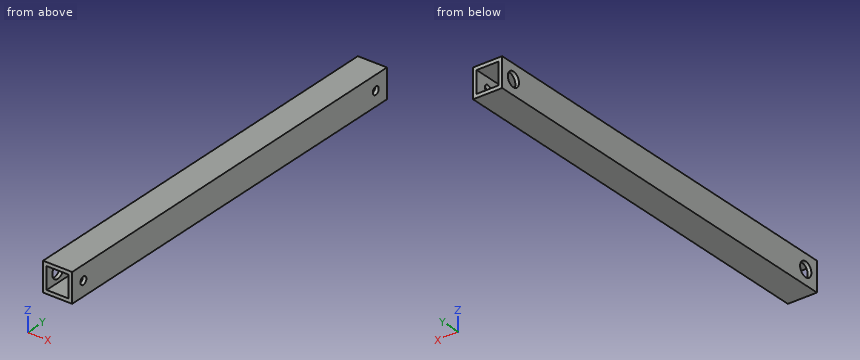
from build123d import *

# Parameters (mm, degrees)
SKETCH1_W           = 25.4
SKETCH1_H           = 25.4
SKETCH1_W_2         = 19.05
SKETCH1_H_2         = 19.05
BOSS_EXTRUDE1_DEPTH = 355.6
SKETCH2_R           = 3.3734375
CUT_EXTRUDE1_DEPTH  = 358.409680899
CUT_EXTRUDE2_REACH  = 359.41
SKETCH3_R           = 6.35


with BuildPart() as part:
    # Sketch1 → Boss-Extrude1 (new body)
    with BuildSketch(Plane(origin=(0, 0, 0), x_dir=(1, 0, 0), z_dir=(0, 1, 0))):
        with Locations((12.7, 12.7)):
            Rectangle(SKETCH1_W, SKETCH1_H)
        with Locations((12.7, 12.7)):
            Rectangle(SKETCH1_W_2, SKETCH1_H_2, mode=Mode.SUBTRACT)
    extrude(amount=BOSS_EXTRUDE1_DEPTH)

    # Sketch2 → Cut-Extrude1 (cut, through all)
    with BuildSketch(Plane(origin=(25.4, 0, 0), x_dir=(0, 0, -1), z_dir=(1, 0, 0))):
        with Locations((12.7, 12.7)):
            Circle(SKETCH2_R)
    cut_extrude1 = extrude(amount=-CUT_EXTRUDE1_DEPTH, mode=Mode.SUBTRACT)

    # Mirror1: Cut-Extrude1 across plane
    add(cut_extrude1.mirror(Plane.ZX.offset(177.8)), mode=Mode.SUBTRACT)

    # Sketch3 → Cut-Extrude2 (cut, up to next)
    with BuildSketch(Plane.ZY, mode=Mode.PRIVATE) as cut_extrude2_sk1:
        with Locations((-12.7, 342.9)):
            Circle(SKETCH3_R)
    cut_extrude2_tool1 = extrude(cut_extrude2_sk1.sketch, amount=-CUT_EXTRUDE2_REACH, mode=Mode.PRIVATE) & part.part
    # Sketch3 → Cut-Extrude2 (cut, up to next)
    with BuildSketch(Plane.ZY, mode=Mode.PRIVATE) as cut_extrude2_sk2:
        with Locations((-12.7, 12.7)):
            Circle(SKETCH3_R)
    cut_extrude2_tool2 = extrude(cut_extrude2_sk2.sketch, amount=-CUT_EXTRUDE2_REACH, mode=Mode.PRIVATE) & part.part
    add(cut_extrude2_tool1.solids().sort_by_distance((0, 342.9, -12.7))[0], mode=Mode.SUBTRACT)
    add(cut_extrude2_tool2.solids().sort_by_distance((0, 12.7, -12.7))[0], mode=Mode.SUBTRACT)


solid = part.part
Work out the finished part from the listing and answer in its coordinate system (mm). Round coordinates to 2 decimals unless told otherwise and drop trailing zeros. Loops run counter-clockwise (first coordinate to the right, second up) from the corner with the lowest first, then second, coordinate; pieces in that order, holes last. Notation, with made-up numbers: (68, -37) -> (81, -37) arc R21 ccw to (81, -7) -> close; hole circle Ø9 at (-2.75, -3). An arc over 180 degrees is marked (long way). Use one line per item in the form item = value.
(1) Find section A-A on x = 6.5. Give the vertices of the cut face in (y, z) (3 decimals).
Answer list:
outline = (0, -25.4) -> (355.6, -25.4) -> (355.6, -22.225) -> (0, -22.225) -> close; (0, -3.175) -> (355.6, -3.175) -> (355.6, 0) -> (0, 0) -> close
(2) A flat-ended cylindrical pin translates along its axis: P1, Ø11.5, axis at y = 12.7, z = -12.7, coming from the -X side (3 decimals). Find the tip coordinate at first contact, or state that the pin passes through.
Answer list:
P1 = 22.225
(3) Find section D-D on y = 283. Give the vertices of the cut face in (x, z) (3 decimals).
Answer list:
outline = (0, -25.4) -> (25.4, -25.4) -> (25.4, 0) -> (0, 0) -> close; hole (3.175, -22.225) -> (22.225, -22.225) -> (22.225, -3.175) -> (3.175, -3.175) -> close
(4) Find section C-C on y = 342.9. Give the vertices of the cut face in (x, z) (3 decimals), then the cut area to 3 significant figures.
Answer list:
outline = (0, -25.4) -> (25.4, -25.4) -> (25.4, -16.073) -> (22.225, -16.073) -> (22.225, -22.225) -> (3.175, -22.225) -> (3.175, -19.05) -> (0, -19.05) -> close; (0, -6.35) -> (3.175, -6.35) -> (3.175, -3.175) -> (22.225, -3.175) -> (22.225, -9.327) -> (25.4, -9.327) -> (25.4, 0) -> (0, 0) -> close
area = 221 mm2
(5) Straight lines are drawn through the part: line 1 (Y direction, x = 23.15, z = -12.7); line 2 (Z direction, x = 21.25, y = 105) (3 decimals); line 3 (Y direction, x = 0.7, z = -12.7). For each, find the intervals that lie inside material, in ascending order.
Answer list:
line_1 = 0 to 9.33, 16.07 to 339.53, 346.27 to 355.6
line_2 = -25.4 to -22.225, -3.175 to 0
line_3 = 0 to 6.35, 19.05 to 336.55, 349.25 to 355.6
(6) Find section B-B on z = -12.7. Give the vertices of the cut face in (x, y) (3 decimals).
Answer list:
outline = (0, 0) -> (3.175, 0) -> (3.175, 6.35) -> (0, 6.35) -> close; (0, 19.05) -> (3.175, 19.05) -> (3.175, 336.55) -> (0, 336.55) -> close; (0, 349.25) -> (3.175, 349.25) -> (3.175, 355.6) -> (0, 355.6) -> close; (22.225, 0) -> (25.4, 0) -> (25.4, 9.327) -> (22.225, 9.327) -> close; (22.225, 16.073) -> (25.4, 16.073) -> (25.4, 339.527) -> (22.225, 339.527) -> close; (22.225, 346.273) -> (25.4, 346.273) -> (25.4, 355.6) -> (22.225, 355.6) -> close
